For this review, use the dimensioned drawing (mm, ordinates from the lowest corner) and the shaded views. A direction names the side the tool comes from. Give positions to 0.01 mm unless a question says otherwise; leave off trailing zeros. Write each loop counter-clockwise with the first axis right and the second up, starting at its lowest first coordinate (ties: lowest second). Pieces come first, ordered by that corner, then holes. Notation, with made-up numbers: (39, 37.25) - (91, 37.25) arc R30 cw to (91, 73.25) - close; hole circle Ø2 at (-19.5, -36.5). An arc over 180 degrees is marked (long way). One line per question, with ' | ' between items. Start each with the question number.
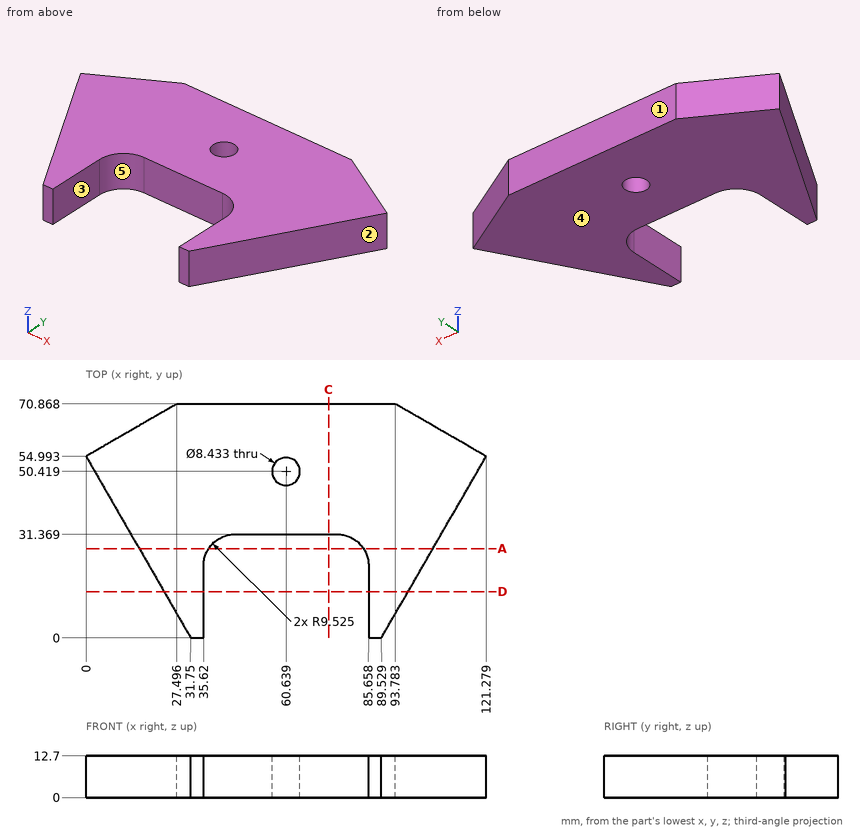
Item 1: Clearance check with flat-ended pins moving along their axes: P1, Ø4, axis at y = 12.5, z = 9, coming from the -X side; P2, Ø1.5, axis at y = 10.5, z = 2, coming from the -X side (1 decimal); P3, Ø6.5, axis at x = 60.64, y = 50.42, coming from the +Z side; P4, Ø1, axis at x = 103.5, z = 8.5, coming from the -Y side (1 decimal). State where each tip first meets the part, or that it passes through.
Item 2: Machinability: for the marked faces 4 and 5, which of the approach directions +Z, -Z, +X, -X, +Y, -Y give a long, thin tool a straight path to every point of the face, cutting with its end or side? Answer none if there is none.
Item 3: Take a section at D-D (y = 14). Give the boundary of the cut face in (x, z).
Item 4: Take a section at C-C (x = 73.5). Give the boundary of the cut face in (y, z), plus the area to 3 significant figures.
Item 5: For probe 1 along X at (y, z) = (23, 8.25); probe 2 along X at (y, z) = (49.5, 1.5) (1 decimal); probe 3 along Y at (x, z) = (51, 9.5), list the stretches that pass through material, from the lowest coordinate up.
Item 6: Take a section at A-A (y = 27). Give the boundary of the cut face in (x, z), plus the area to 3 significant figures.
Item 7: The part is to be moulded in two halves that separate along X. For the marked faces 1, 2 and 3, say which applies: +X half, -X half, draft (parallel to the pull), parting line (faces both ways), or undercut.
Check sheet entries:
1) P1: stops at x = 23.38 | P2: stops at x = 25.3 | P3: passes through | P4: stops at y = 23.3
2) face 4: -Z, +X, -X, +Y, -Y | face 5: +Z, -Z, -Y
3) outline: (23.67, 0) - (35.62, 0) - (35.62, 12.7) - (23.67, 12.7) - close; (85.66, 0) - (97.61, 0) - (97.61, 12.7) - (85.66, 12.7) - close
4) outline: (31.37, 0) - (70.87, 0) - (70.87, 12.7) - (31.37, 12.7) - close | area: 502 mm^2
5) probe 1: x = 18.47 to 35.69, 85.59 to 102.81 | probe 2: x = 3.2 to 56.5, 64.8 to 118.1 | probe 3: y = 31.37 to 70.87
6) outline: (16.16, 0) - (37.14, 0) - (37.14, 12.7) - (16.16, 12.7) - close; (84.14, 0) - (105.12, 0) - (105.12, 12.7) - (84.14, 12.7) - close | area: 533 mm^2
7) face 1: draft | face 2: +X half | face 3: undercut
